```python
from build123d import *

# Parameters (mm, degrees)
BOSS_EXTRUDE1_DEPTH     = 4
SKETCH1_3_W             = 12
SKETCH1_3_H             = 12
BOSS_EXTRUDE2_DEPTH     = 19
BOSS_EXTRUDE3_DEPTH     = 7
BOSS_EXTRUDE4_START     = 19
SKETCH1_6_W             = 2
SKETCH1_6_H             = 5
BOSS_EXTRUDE4_DEPTH     = 2
BOSS_EXTRUDE5_DEPTH     = 12
BOSS_EXTRUDE6_DEPTH     = 4
SKETCH5_R               = 1.5
SKETCH5_W               = 5
SKETCH5_H               = 1
CUT_EXTRUDE1_DEPTH      = 73.739260376
CUT_EXTRUDE2_DEPTH      = 71.334913094
CUT_EXTRUDE2_DEPTH_BACK = 9
SKETCH6_R               = 2
SKETCH7_R               = 3.5
SKETCH7_R_2             = 2
CUT_EXTRUDE3_DEPTH      = 69.607579756
CUT_EXTRUDE4_DEPTH      = 2
CHAMFER1_SIZE           = 2


with BuildPart() as part:
    # Sketch1 → Boss-Extrude1 (new body)
    with BuildSketch(Plane(origin=(0, 0, 0), x_dir=(1, 0, 0), z_dir=(0, 1, 0))):
        with BuildLine():
            Line((33, 5), (33, 6))
            Line((33, 6), (0, 6))
            Line((0, 6), (0, 0))
            Line((0, 0), (3.5, 0))
            ThreePointArc((3.5, 0), (7, 3.5), (10.5, 0))
            Line((10.5, 0), (33, 0))
            Line((33, 0), (33, 5))
        make_face()
        with BuildLine():
            Line((33, -5), (33, 0))
            Line((33, 0), (10.5, 0))
            ThreePointArc((10.5, 0), (7, -3.5), (3.5, 0))
            Line((3.5, 0), (0, 0))
            Line((0, 0), (0, -6))
            Line((0, -6), (33, -6))
            Line((33, -6), (33, -5))
        make_face()
    extrude(amount=BOSS_EXTRUDE1_DEPTH)

    # Sketch1<3> → Boss-Extrude2 (add)
    with BuildSketch(Plane(origin=(0, 0, 0), x_dir=(1, 0, 0), z_dir=(0, 1, 0))):
        with Locations((39, 0)):
            Rectangle(SKETCH1_3_W, SKETCH1_3_H)
    extrude(amount=BOSS_EXTRUDE2_DEPTH)

    # Sketch1<4> → Boss-Extrude3 (add)
    with BuildSketch(Plane(origin=(0, 0, 0), x_dir=(1, 0, 0), z_dir=(0, 1, 0))):
        Polygon((65, -2), (45, -2), (45, -5), (45, -6), (65, -6), align=None)
    extrude(amount=BOSS_EXTRUDE3_DEPTH)

    # Sketch1<6> → Boss-Extrude4 (add)
    with BuildSketch(Plane(origin=(0, 0, 0), x_dir=(1, 0, 0), z_dir=(0, 1, 0)).offset(BOSS_EXTRUDE4_START)):
        with Locations((34, -2.5)):
            Rectangle(SKETCH1_6_W, SKETCH1_6_H)
        with Locations((34, 2.5)):
            Rectangle(SKETCH1_6_W, SKETCH1_6_H)
        Polygon((45, -2), (45, 0), (43, 0), (43, -5), (45, -5), align=None)
        with Locations((44, 2.5)):
            Rectangle(SKETCH1_6_W, SKETCH1_6_H)
    extrude(amount=BOSS_EXTRUDE4_DEPTH)

    # Sketch2 → Boss-Extrude5 (add)
    with BuildSketch(Plane(origin=(0, 7, 0), x_dir=(1, 0, 0), z_dir=(0, 1, 0))):
        Polygon((45, -6), (45, 15), (65, 15), (65, -6), (61, -6), (61, 11), (49, 11), (49, -6), align=None)
    extrude(amount=BOSS_EXTRUDE5_DEPTH)

    # Sketch4 → Boss-Extrude6 (add)
    with BuildSketch(Plane(origin=(0, 0, -15), x_dir=(-1, 0, 0), z_dir=(0, 0, -1))):
        with BuildLine():
            ThreePointArc((-51.5, 13), (-54.065732463, 16.373002249), (-58.00122524, 14.800735144))
            Line((-58.00122524, 14.800735144), (-51.99877476, 11.199264856))
            ThreePointArc((-51.99877476, 11.199264856), (-51.626997751, 12.065732463), (-51.5, 13))
        make_face()
        with BuildLine():
            Line((-51.99877476, 11.199264856), (-58.00122524, 14.800735144))
            ThreePointArc((-58.00122524, 14.800735144), (-56.800735144, 9.99877476), (-51.99877476, 11.199264856))
        make_face()
    extrude(amount=BOSS_EXTRUDE6_DEPTH)

    # Sketch5 → Cut-Extrude1 (cut, through all)
    with BuildSketch(Plane.XY.offset(6)):
        with Locations((55, 4)):
            Circle(SKETCH5_R)
        with Locations((55, 6.5)):
            Rectangle(SKETCH5_W, SKETCH5_H)
    extrude(amount=-CUT_EXTRUDE1_DEPTH, mode=Mode.SUBTRACT)

    # Sketch6 → Cut-Extrude2 (cut, two sides: drawn at the far end of the back side and taken through both)
    with BuildSketch(Plane(origin=(0, 19, 0), x_dir=(1, 0, 0), z_dir=(0, 1, 0)).offset(-CUT_EXTRUDE2_DEPTH_BACK)):
        with Locations(Location((39, 0, 0), (0, 0, 270))):
            Circle(SKETCH6_R)
    extrude(amount=CUT_EXTRUDE2_DEPTH + CUT_EXTRUDE2_DEPTH_BACK, mode=Mode.SUBTRACT)

    # Sketch7 → Cut-Extrude3 (cut, through all)
    # profile 1 of 2: a face of its own
    with BuildSketch(Plane(origin=(0, 10, 0), x_dir=(1, 0, 0), z_dir=(0, 1, 0))):
        with Locations(Location((39, 0, 0), (0, 0, 270))):
            Circle(SKETCH7_R)
        with Locations(Location((39, 0, 0), (0, 0, 270))):
            Circle(SKETCH7_R_2, mode=Mode.SUBTRACT)
    # profile 2 of 2: a face of its own
    with BuildSketch(Plane(origin=(0, 10, 0), x_dir=(1, 0, 0), z_dir=(0, 1, 0))):
        with Locations(Location((39, 0, 0), (0, 0, 270))):
            Circle(SKETCH7_R_2)
    extrude(amount=-CUT_EXTRUDE3_DEPTH, mode=Mode.SUBTRACT)

    # Sketch8 → Cut-Extrude4 (cut)
    with BuildSketch(Plane.XZ):
        with BuildLine():
            Line((31.125, 1.996089928), (7.21875, 3.493157374))
            ThreePointArc((7.21875, 3.493157374), (9.551041454, 2.396286189), (10.5, 0))
            ThreePointArc((10.5, 0), (9.551041454, -2.396286189), (7.21875, -3.493157374))
            Line((7.21875, -3.493157374), (31.125, -1.996089928))
            ThreePointArc((31.125, -1.996089928), (33, 0), (31.125, 1.996089928))
        make_face()
    extrude(amount=-CUT_EXTRUDE4_DEPTH, mode=Mode.SUBTRACT)

    # Chamfer1
    chamfer1_edges = [part.edges().sort_by_distance(p)[0] for p in [
        (0, 2, -6),
        (0, 2, 6),
    ]]
    chamfer(chamfer1_edges, length=CHAMFER1_SIZE)


solid = part.part
```
Build history of the part. All positions in model axes, mm. A direction names the side the tool comes from. Round coordinates to 2 decimals unless told otherwise and drop trailing zeros. Write each loop counter-clockwise with the first axis right and the second up, starting at its lowest first coordinate (ties: lowest second). Pieces come first, ordered by that corner, then holes. Notation, with made-up numbers: (58, 51.25) - (109, 51.25) arc R28 cw to (109, 77.25) - close; hole circle Ø5 at (-33.75, -11). An arc over 180 degrees is marked (long way). Write each question's results on one line, items separated by ' | '. Start each with the question number.
Item 1: Saw through at C-C (z = -8.75). Write the cut outline in (x, y).
Item 2: Which spindle directions (+Z, -Z, +X, -X, +Y, -Y) get a long thin tool onto all of the face, cutting with end or side? Do faces 1 (the face through (45, 13, -10)), 2 (the face through (35, 20, 0)), 3 (the face through (49, 13, -3)), 4 (the face through (45, 20, 0)), 5 (the face through (20, 2, 0)). Say none if no direction does.
Item 3: Saw through at B-B (y = 8.5). Write the cut outline in (x, z), and give its area (3 significant figures).
Item 4: Wall check: L1, parallel to X at y = 16.25, z = 0; L2, parallel to Z at x = 39, y = 15.5; L3, parallel to X at y = 20.25, z = -1.5. Give the ranges that are in metal, low to high. Write a range as [from, to].
Item 5: Saw through at A-A (z = 0). State how many separate pieces and enclosed holes the cut face has, and give its area (3 significant figures).
Item 6: Mould opens along Z. For faces 6 (the face through (33, 1, 0)), 7 (the face through (43, 20, 0)), 8 (the face through (55, 13, -19)) say: pulls with the +Z half, pulls with the -Z half, needs draft (parallel to the pull), parting line crosses it, or undercut.
Item 7: Drop flat-ended pins along their axis: P1, Ø6, axis at x = 28.5, y = 10, coming from the +Z side; P2, Ø2, axis at x = 39.5, z = -1, coming from the -Y side; P3, Ø3.5, axis at x = 52.5, y = 12, coming from the +Z side; P4, Ø5, axis at x = 38.5, z = -3.5, coming from the +Y side. Give the stop position or say it passes through.
Item 8: Saw through at D-D (x = 46). Write the cut outline in (y, z), and give its area (3 significant figures).
Results are:
1) outline: (45, 7) - (49, 7) - (49, 19) - (45, 19) - close; (61, 7) - (65, 7) - (65, 19) - (61, 19) - close
2) face 1: -Z, -X, +Y, -Y | face 2: +Z, -Z, +Y | face 3: +Z, +Y | face 4: +Z, -Z, +X, +Y | face 5: -Y
3) outline: (33, -6) - (45, -6) - (45, -15) - (65, -15) - (65, 6) - (61, 6) - (61, -11) - (49, -11) - (49, 6) - (33, 6) - close; hole circle Ø7 at (39, 0) | area: 322 mm²
4) L1: x = [33, 37], [41, 49], [61, 65] | L2: z = [-6, -2], [2, 6] | L3: x = [33, 35], [43, 45]
5) separate pieces: 4 | enclosed holes: 0 | area: 285 mm²
6) face 6: undercut | face 7: needs draft | face 8: pulls with the -Z half
7) P1: passes through | P2: stops at y = 10 | P3: stops at z = -11 | P4: stops at y = 19
8) outline: (0, 2) - (7, 2) - (7, -15) - (19, -15) - (19, 6) - (0, 6) - close | area: 280 mm²
